Model file for the job. Use its own axes, mm. Give positions to 0.01 mm unless a question says otherwise; leave off trailing zeros. Write each loop counter-clockwise with the first axis right and the second up, starting at its lowest first coordinate (ties: lowest second). Pieces come first, ordered by that corner, then holes. Notation, with made-up numbers: (42.25, 48.25) - (46.25, 48.25) arc R22 cw to (46.25, 74.25) - close; hole circle Ø3 at (-14, -1). An arc over 180 degrees is marked (long way). Use a Markdown table: item, result. Add a question column.
```python
from build123d import *

# Parameters (mm, degrees)
SKETCH1_R           = 1.27
BOSS_EXTRUDE1_DEPTH = 3.175


with BuildPart() as part:
    # Sketch1 → Boss-Extrude1 (new body)
    with BuildSketch(Plane(origin=(0, 0, 0), x_dir=(1, 0, 0), z_dir=(0, 1, 0))):
        Polygon((0, 0), (-51.450921593, 21.881601753), (-63.876832212, -7.335845865), (-14.324041053, -28.410190275), (0, -28.410190275), align=None)
        with Locations(Location((-49.899383574, 18.033755451, 0), (0, 0, 270))):
            Circle(SKETCH1_R, mode=Mode.SUBTRACT)
        with Locations(Location((-60.028985911, -5.784307846, 0), (0, 0, 270))):
            Circle(SKETCH1_R, mode=Mode.SUBTRACT)
        with Locations(Location((-17.257741053, -23.974523249, 0), (0, 0, 270))):
            Circle(SKETCH1_R, mode=Mode.SUBTRACT)
        with Locations(Location((-7.128138716, -0.156459951, 0), (0, 0, 270))):
            Circle(SKETCH1_R, mode=Mode.SUBTRACT)
    extrude(amount=BOSS_EXTRUDE1_DEPTH)


solid = part.part
```
(1) Flat gauge pins, fed straight in: pin 1 (2 mm diameter, centred on x = -57, z = 12, fed in from -Y); pin 2 (1 mm diameter, centred on x = -52.5, y = 2.5, fed in from +Z). Where does each tip first touch, or does it go through?
(2) Band-saw the part on B-B (y = 1.05). Write the cut outline in (x, z).
(3) Band-saw the part on A-A (z = 23.5). Write the cut outline in (x, y) (3 decimals).
(4) Band-saw the part on D-D (z = -13). Write the cut outline in (x, y) (3 decimals), then the cut area to 3 significant figures.
(5) Two-plate mould, pull along X, no slides. Class faces 1 (the flat face through (-32, 0, 3)), 2 (the cylindrical face through (-16.19, 1.57, 24.66)), 3 (the flat face through (-39.447, 1.565, 17.725)): +X half, -X half, draft (parallel to the pull), parting line (faces both ways), or undercut.
(6) Band-saw the part on C-C (x = -55). Write the cut outline in (y, z) (3 decimals).
(7) Probe probe 1 along X at (y, z) = (2.15, 0.5); probe 2 along Z at (x, y) = (-59, 0.25); probe 3 along X at (y, z) = (2.95, -18). List the from-to ranges inside material, lowest first. Write a range as [from, to].
Model answer:
| question | item | result |
|---|---|---|
| 1 | pin 1 | passes through |
| 1 | pin 2 | stops at z = 12.39 |
| 2 | outline | (-63.88, 7.34) - (-51.45, -21.88) - (0, 0) - (0, 28.41) - (-14.32, 28.41) - close; hole circle Ø2.54 at (-60.03, 5.78); hole circle Ø2.54 at (-49.9, -18.03); hole circle Ø2.54 at (-17.26, 23.97); hole circle Ø2.54 at (-7.13, 0.16) |
| 3 | outline | (-25.87, 0) - (-18.436, 0) - (-18.436, 3.175) - (-25.87, 3.175) - close; (-16.08, 0) - (0, 0) - (0, 3.175) - (-16.08, 3.175) - close |
| 4 | outline | (-55.228, 0) - (-30.567, 0) - (-30.567, 3.175) - (-55.228, 3.175) - close |
| 4 | area | 78.3 mm^2 |
| 5 | face 1 | draft |
| 5 | face 2 | undercut |
| 5 | face 3 | -X half |
| 6 | outline | (0, -13.537) - (3.175, -13.537) - (3.175, 11.111) - (0, 11.111) - close |
| 7 | probe 1 | x = [-60.97, -8.35], [-5.91, 0] |
| 7 | probe 2 | z = [-4.13, 5.04], [6.53, 9.41] |
| 7 | probe 3 | x = [-53.1, -51.17], [-48.63, -42.32] |
